from build123d import *

# Parameters (mm, degrees)
F0_R     = 2.15
F1_DEPTH = 15
F3_D     = 5.5
F4_SIZE  = 0.5
F6_D     = 3
F6_DEPTH = 3
F6_TIP   = 0.9012909285
F8_D     = 3
F8_DEPTH = 3
F8_TIP   = 0.9012909285


with BuildPart() as f1:
    # F0 (on Front) → F1 (new body)
    with BuildSketch(Plane.XZ):
        with BuildLine():
            Line((-12.5, 4.5), (-12.5, 0))
            Line((-12.5, 0), (0, 0))
            Line((0, 0), (12.5, 0))
            Line((12.5, 0), (12.5, 4.5))
            ThreePointArc((12.5, 4.5), (8.7106121428, 8.9589284982), (3.6988942602, 5.9383014856))
            ThreePointArc((3.6988942602, 5.9383014856), (2.8137586471, 4.8915084722), (1.5, 4.5))
            Line((1.5, 4.5), (0, 4.5))
            Line((0, 4.5), (-1.5, 4.5))
            ThreePointArc((-1.5, 4.5), (-2.8137586471, 4.8915084722), (-3.6988942602, 5.9383014856))
            ThreePointArc((-3.6988942602, 5.9383014856), (-8.7106121428, 8.9589284982), (-12.5, 4.5))
        make_face()
        with Locations((-7.9819214904, 4.5)):
            Circle(F0_R, mode=Mode.SUBTRACT)
        with Locations((7.9819214904, 4.5)):
            Circle(F0_R, mode=Mode.SUBTRACT)
    extrude(amount=F1_DEPTH)

    # F3 (through all)
    with Locations(Plane(origin=(0, 0, 0), x_dir=(1, 0, 0), z_dir=(0, 0, -1))):
        with Locations((0, 6.5)):
            Hole(F3_D / 2)

    # F4
    f4_edges = [f1.edges().sort_by_distance(p)[0] for p in [
        (-10.131921, 0, 4.5),
        (5.831921, 0, 4.5),
        (-10.131921, -15, 4.5),
        (5.831921, -15, 4.5),
        (-2.75, -6.5, 0),
    ]]
    chamfer(f4_edges, length=F4_SIZE)

    # F6
    with Locations(Plane(origin=(-12.5, 0, 0), x_dir=(0, -1, 0), z_dir=(-1, 0, 0))):
        with Locations((7.5, 4.5)):
            Hole(F6_D / 2, depth=F6_DEPTH)
            with Locations((0, 0, -(F6_DEPTH + F6_TIP / 2))):  # 118° drill point
                Cone(0, F6_D / 2, F6_TIP, mode=Mode.SUBTRACT)

    # F8
    with Locations(Plane.YZ.offset(12.5)):
        with Locations((-7.5, 4.5)):
            Hole(F8_D / 2, depth=F8_DEPTH)
            with Locations((0, 0, -(F8_DEPTH + F8_TIP / 2))):  # 118° drill point
                Cone(0, F8_D / 2, F8_TIP, mode=Mode.SUBTRACT)


solid = f1.part
Work out the finished part from the listing and answer in its coordinate system (mm). A direction names the side the tool comes from. Coordinates: 2 decimals unless noted, no trailing zeros. Write each loop counter-clockwise with the first axis right and the second up, starting at its lowest first coordinate (ties: lowest second). Pieces come first, ordered by that corner, then holes. Notation, with made-up numbers: M 41.5,-35.5 L 76.5,-35.5 A29 cw 76.5,-5.5 Z; hole C 68,0 d1. An arc over 180 degrees is marked long. Answer as CSV lines item,"result". Start each with the question number.
Item 1: Section C-C on y = -6.5 is taken. Write down the section's boundary in (x, z), and give its area (3 significant figures).
Item 2: Section D-D on z = 3.25 is taken. Give the number of separate pieces and of enclosed holes in the cut face, and give its area (3 significant figures).
Item 3: Flat-ended cylindrical pins translate along their axes: P1, Ø5, axis at x = 8.5, y = -8, coming from the -Z side; P2, Ø2, axis at x = 1, y = -11.5, coming from the +Z side; P3, Ø2.5, axis at y = -7.5, z = 4.5, coming from the +X side; P4, Ø1, axis at x = 6.5, y = -12.5, coming from the +Z side. Find the tip coordinate at first contact, or state that the pin passes through.
Item 4: Section B-B on x = 0 is taken. Write down the section's boundary in (y, z), and give its area (3 significant figures).
Item 5: Determine the mould class of faces 3 (the face through (0, 0, 4)), 4 (the face through (5.834, -7.402, 4.595)), 5 (the face through (0, -15, 4)), 6 (the face through (11, -6.3, 3.6)) for opening direction Y: released by +Y, released by -Y, zero draft, split by the parting line, or undercut.
Item 6: Section A-A on y = -10.25 is taken. Write down the section's boundary in (x, z), and give its area (3 significant figures).
Item 7: A tool of negligible diameter and unlimited length cuts with its end or side. For faces 1 (the face through (-2.797, -7.395, 4.881)), 2 (the face through (-3, -9, 0)), from which of +Z, -Z, +X, -X, +Y, -Y can it reach the whole face along a straight path? Write none if from no direction.
Item 8: Consider L1, parallel to Y at x = 0, z = 3.6; L2, parallel to X at y = -6.5, z = 2.7; L3, parallel to X at y = -13, z = 6.25. Determine where each line is inside the solid, lowest interval first.
Checks:
1,outline,"M -12.5,0 L -3.25,0 L -2.75,0.5 L -2.75,4.85 A2.4 cw -3.7,5.94 A4.52 ccw -12.36,5.62 L -9.82,5.62 A2.15 cw long -9.82,3.38 L -12.5,3.38 Z; M 2.75,0.5 L 3.25,0 L 12.5,0 L 12.5,3.38 L 9.82,3.38 A2.15 cw long 9.82,5.62 L 12.36,5.62 A4.52 ccw 3.7,5.94 A2.4 cw 2.75,4.85 Z"
1,area,"113 mm²"
2,separate pieces,"5"
2,enclosed holes,"1"
2,area,"236 mm²"
3,P1,"stops at z = 0"
3,P2,"stops at z = 4.55"
3,P3,"stops at x = 6.23"
3,P4,"stops at z = 8.91"
4,outline,"M -15,0 L -9.75,0 L -9.25,0.5 L -9.25,4.5 L -15,4.5 Z; M -3.75,0.5 L -3.25,0 L 0,0 L 0,4.5 L -3.75,4.5 Z"
4,area,"42.5 mm²"
5,face 3,"released by +Y"
5,face 4,"zero draft"
5,face 5,"released by -Y"
5,face 6,"undercut"
6,outline,"M -12.5,0 L 12.5,0 L 12.5,4.5 A4.52 ccw 3.7,5.94 A2.4 cw 1.5,4.5 L -1.5,4.5 A2.4 cw -3.7,5.94 A4.52 ccw -12.5,4.5 Z; hole C -7.98,4.5 d4.3; hole C 7.98,4.5 d4.3"
6,area,"149 mm²"
7,face 1,"+Z, +Y, -Y"
7,face 2,"-Z, +X, -X, +Y, -Y"
8,L1,"y = -15 to -9.25, -3.75 to 0"
8,L2,"x = -12.5 to -9.16, -6.81 to -2.75, 2.75 to 6.81, 9.16 to 12.5"
8,L3,"x = -12.15 to -9.23, -6.73 to -3.82, 3.82 to 6.73, 9.23 to 12.15"
